Input: part model. Units: mm. Frame: model coordinates. Face numbers are marked on the shaded views. Round coordinates to 2 decimals unless told otherwise and drop trailing zeros. Loops run counter-clockwise (first coordinate to the right, second up) from the corner with the lowest first, then second, coordinate; pieces in that order, holes last. Notation, with made-up numbers: (19, -35.75) -> (34, -35.75) arc R29 cw to (34, -9.75) -> close; hole circle Ø7 at (82, 23.5). An arc over 180 degrees is marked (long way). Answer in a Markdown table with one row per item. Add a question column.
Q1. Ray query, L1, parallel to X at y = 57, z = 0.25; L2, parallel to Z at x = 3.5, y = 56.5; L3, parallel to X at y = 59, z = -2.25. Return the intervals inside material, ascending. Write a range as from..to.
Q2. Section C-C, the plane y = 30.5. Output: boundary loops of the cut face in (x, z).
Q3. Section A-A, the plane z = 0. Output: boundary loops of the cut face in (x, y), and give its area (3 significant figures).
Q4. Mould query, pull axis Y, two halves, no side actions, for the marked faces 1, 2 and 3. Classes: pulls with the +Y half, pulls with the -Y half, needs draft (parallel to the pull), parting line crosses it, or undercut.
Q5. Section B-B, the plane x = 0. Output: boundary loops of the cut face in (y, z), and give its area (3 significant figures).
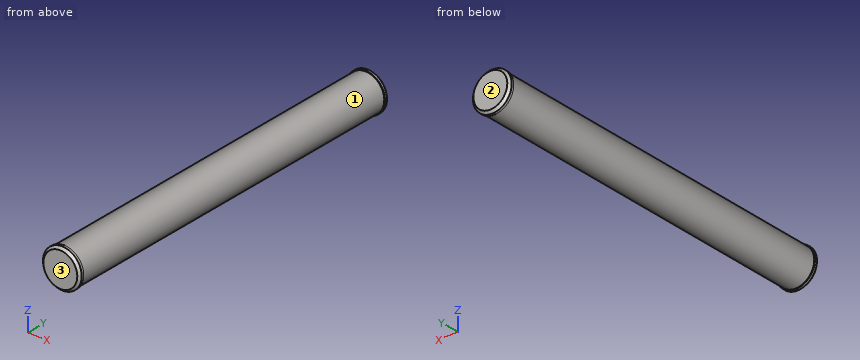
```python
from build123d import *

# Parameters (mm, degrees)
SKETCH_1_R      = 3.85
EXTRUDE_1_DEPTH = 75
SKETCH_3_R      = 4
EXTRUDE_2_DEPTH = 1
EXTRUDE_START   = 1
SKETCH_4_R      = 4
EXTRUDE_3_DEPTH = 1
CHAMFER_1_SIZE  = 0.5


with BuildPart() as part:
    # 草图1 → 凸台-拉伸1 (new body)
    with BuildSketch(Plane(origin=(0, 0, 0), x_dir=(1, 0, 0), z_dir=(0, 1, 0))):
        with Locations(Location((0, 0, 0), (0, 0, 270))):
            Circle(SKETCH_1_R)
    extrude(amount=EXTRUDE_1_DEPTH)

    # 草图3 → 凸台-拉伸2 (add)
    with BuildSketch(Plane(origin=(0, 75, 0), x_dir=(1, 0, 0), z_dir=(0, 1, 0))):
        with Locations(Location((0, 0, 0), (0, 0, 270))):
            Circle(SKETCH_3_R)
    extrude(amount=EXTRUDE_2_DEPTH)

    # 草图4 → 凸台-拉伸3 (add)
    with BuildSketch(Plane.XZ.offset(EXTRUDE_START)):
        with Locations(Location((0, 0, 0), (0, 0, 90))):
            Circle(SKETCH_4_R)
    extrude(amount=-EXTRUDE_3_DEPTH)

    # 倒角1
    chamfer_1_edges = [part.edges().sort_by_distance(p)[0] for p in [
        (0, -1, -4),
        (0, 76, -4),
    ]]
    chamfer(chamfer_1_edges, length=CHAMFER_1_SIZE)


solid = part.part
```
Answer block:
| question | item | result |
|---|---|---|
| 1 | L1 | -3.84..3.84 |
| 1 | L2 | -1.6..1.6 |
| 1 | L3 | -3.12..3.12 |
| 2 | outline | circle Ø7.7 at (0, 0) |
| 3 | outline | (-4, -0.5) -> (-3.5, -1) -> (3.5, -1) -> (4, -0.5) -> (4, 0) -> (3.85, 0) -> (3.85, 75) -> (4, 75) -> (4, 75.5) -> (3.5, 76) -> (-3.5, 76) -> (-4, 75.5) -> (-4, 75) -> (-3.85, 75) -> (-3.85, 0) -> (-4, 0) -> close |
| 3 | area | 593 mm^2 |
| 4 | face 1 | undercut |
| 4 | face 2 | pulls with the +Y half |
| 4 | face 3 | pulls with the -Y half |
| 5 | outline | (-1, -3.5) -> (-0.5, -4) -> (0, -4) -> (0, -3.85) -> (75, -3.85) -> (75, -4) -> (75.5, -4) -> (76, -3.5) -> (76, 3.5) -> (75.5, 4) -> (75, 4) -> (75, 3.85) -> (0, 3.85) -> (0, 4) -> (-0.5, 4) -> (-1, 3.5) -> close |
| 5 | area | 593 mm^2 |
